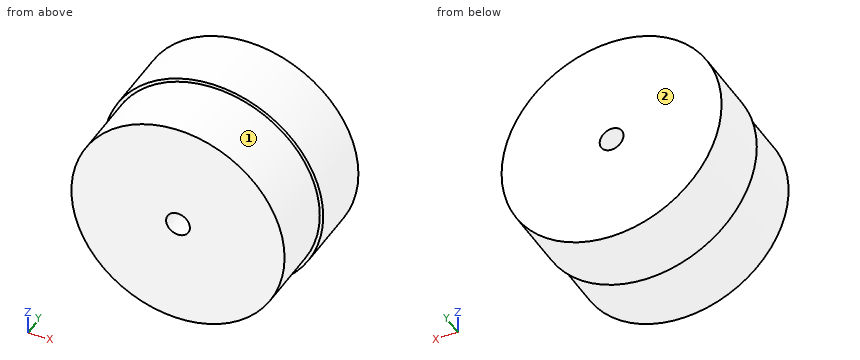
Autodesk Inventor part; units mm, degrees
ref_plane "YZ Plane" through (0, 0, 0) normal (1, 0, 0) x (0, 1, 0)
ref_plane "XZ Plane" through (0, 0, 0) normal (0, 1, 0) x (-1, 0, 0)
ref_plane "XY Plane" through (0, 0, 0) normal (0, 0, 1) x (1, 0, 0)
sketch "Sketch4" plane through (0, 0, 0) normal (0, 1, 0) x (-1, 0, 0)
  circle A0 centre (0, 0) radius 16
  dimension "d19" = 32
extrude "Extrusion2" add sketch "Sketch4" along normal blind 10
sketch "Sketch5" plane through (0, 0, 0) normal (0, -1, 0) x (1, 0, 0)
  circle A0 centre (0, 0) radius 15.5
  dimension "d22" = 31
extrude "Extrusion3" add sketch "Sketch5" along normal blind 10
sketch "Sketch6" plane through (0, 10, 0) normal (0, 1, 0) x (1, 0, 0)
  point P0 (0, 0)
  point P1 (0, 0)
hole "Hole2" at (0, 10, 0) direction (0, -1, 0) diameter 3.4587 end through all
equation "\"d30\" = Thickness"
equation "\"BendRadius\" = Thickness"
equation "\"BendReliefWidth\" = Thickness"
equation "\"BendReliefDepth\" = 0.5 * Thickness"
equation "\"CornerReliefSize\" = 4 * Thickness"
equation "\"MinimumRemnant\" = 2 * Thickness"
equation "\"TransitionRadius\" = BendRadius"
equation "\"JacobiRadiusSize\" = BendRadius"
equation "\"GapSize\" = Thickness"
properties part number "Output link probe hub_ final"
Geometry check sheet. Reference: the model listing, model coordinates, mm. Face numbers are marked on the shaded views. A direction names the side the tool comes from. Give positions to 0.01 mm unless a question says otherwise; leave off trailing zeros. Loops run counter-clockwise (first coordinate to the right, second up) from the corner with the lowest first, then second, coordinate; pieces in that order, holes last.
(1) Section check A-A on x = 0. Record the cut outline in (y, z), then the cut area to 3 significant figures.
From the geometry:
outline: (-10, -15.5) - (0, -15.5) - (0, -16) - (10, -16) - (10, -1.73) - (-10, -1.73) - close; (-10, 1.73) - (10, 1.73) - (10, 16) - (0, 16) - (0, 15.5) - (-10, 15.5) - close
area: 561 mm2
(2) Set-up check for the marked faces 1 and 2: record each of +Z, -Z, +X, -X, +Y, -Y from which the full face is reachable in a straight line by a thin tool's end or side.
From the geometry:
face 1: -Y
face 2: +Z, -Z, +X, -X, +Y
(3) Section check C-C on x = -10.5. Record the cut outline in (y, z), then the cut area to 3 significant figures.
From the geometry:
outline: (-10, -11.4) - (0, -11.4) - (0, -12.07) - (10, -12.07) - (10, 12.07) - (0, 12.07) - (0, 11.4) - (-10, 11.4) - close
area: 469 mm2
(4) Section check B-B on y = -6.25. Record the cut outline in (x, z), then the cut area to 3 significant figures.
From the geometry:
outline: circle Ø31 at (0, 0); hole circle Ø3.46 at (0, 0)
area: 745 mm2
(5) Depth check by flat-ended pin: pin 1 Ø10 at (x, y) = (9.5, -0.5) entering from +Z; pin 2 Ø5 at (x, y) = (2, -5) entering from +Z; pin 3 Ø12 at (x, y) = (-10.5, 5.5) entering from +Z. Enter the tip coordinate at first touch or a pass-through.
From the geometry:
pin 1: stops at z = 15.35
pin 2: stops at z = 15.5
pin 3: stops at z = 15.35
(6) Section check D-D on z = 3. Record the cut outline in (x, y).
From the geometry:
outline: (-15.72, 0) - (-15.21, 0) - (-15.21, -10) - (15.21, -10) - (15.21, 0) - (15.72, 0) - (15.72, 10) - (-15.72, 10) - close
(7) Thickness scan on L1, parallel to Z at x = 0, y = 4.25; L2, parallel to Z at x = 0, y = -4.25; L3, parallel to Z at x = -13, y = 0.25. Record the ranges inside material, lowest first.
From the geometry:
L1: z = -16 to -1.73, 1.73 to 16
L2: z = -15.5 to -1.73, 1.73 to 15.5
L3: z = -9.33 to 9.33
